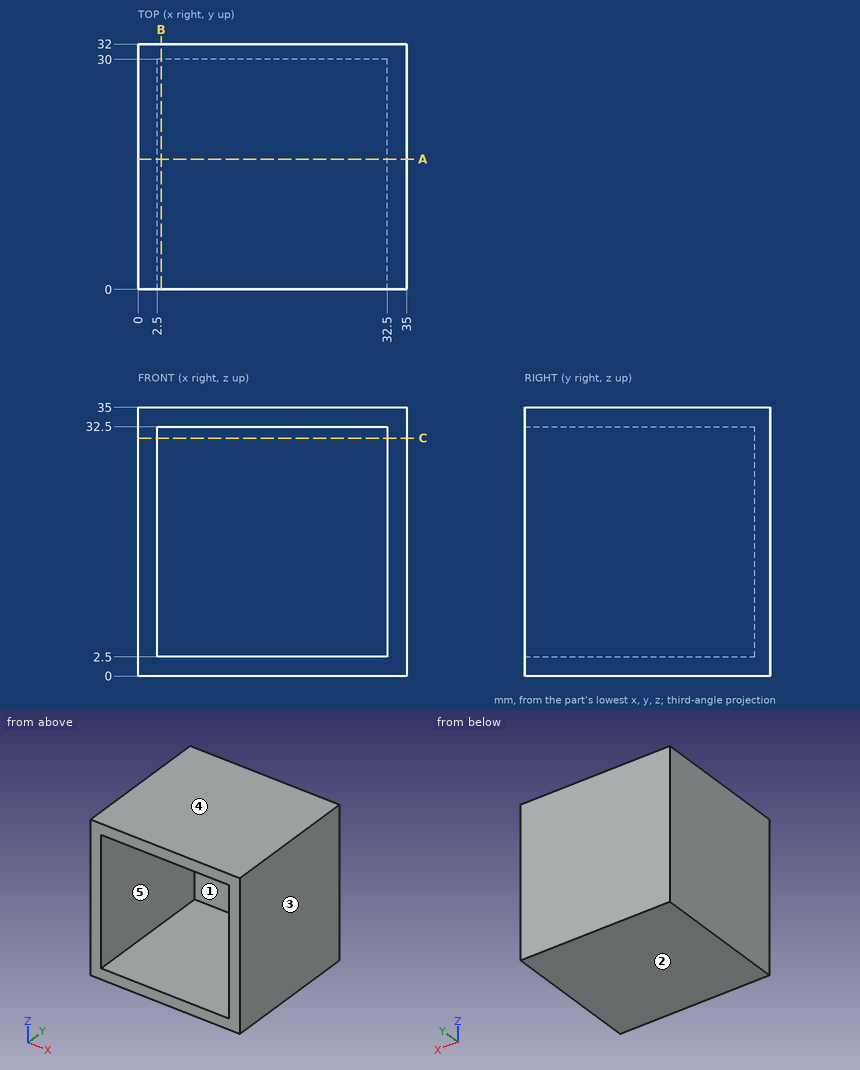
For this review, use the dimensioned drawing (mm, ordinates from the lowest corner) and the shaded views. A direction names the side the tool comes from. Give positions to 0.01 mm unless a question says otherwise; leave off trailing zeros. Write each loop counter-clockwise with the first axis right and the second up, starting at its lowest first coordinate (ties: lowest second). Pieces come first, ordered by that corner, then holes. Notation, with made-up numbers: M 88.5,80 L 146.5,80 A35 ccw 146.5,118 Z; hole C 52.25,61 d3. An arc over 180 degrees is marked long. Answer as a JSON object with one key per item and string values. Group by question number.
1) We need section C-C (z = 31). Give the boundary of the cut face in (x, y), and give its area (3 significant figures).
2) We need section A-A (y = 17). Give the boundary of the cut face in (x, z), and give its area (3 significant figures).
3) We need section B-B (x = 3). Give the boundary of the cut face in (y, z), and give its area (3 significant figures).
4) Mouldability with a two-part tool opening along Z and no side actions: class the marked faces 3, 4 and 5 as released by +Z, released by -Z, zero draft, split by the parting line, or undercut.
5) For line 1 along X through (y, z) = (5, 3.5); line 2 along Y through (x, z) = (22.5, 27), list the stretches that pass through material, from the lowest coordinate up.
6) Tool access review of the marked faces 1 and 2: name each direction out of +Z, -Z, +X, -X, +Y, -Y from which nothing blocks a thin tool from reaching the whole face with its end or side.
7) Clearance check with a flat-ended pin moving along its axis: pin 1 Ø15 at (x, z) = (24, 13.5) entering from -Y. State where the tip first meets the part, or that it passes through.
Answer key:
{
 "1": {"outline": "M 0,0 L 2.5,0 L 2.5,30 L 32.5,30 L 32.5,0 L 35,0 L 35,32 L 0,32 Z", "area": "220 mm²"},
 "2": {"outline": "M 0,0 L 35,0 L 35,35 L 0,35 Z; hole M 2.5,2.5 L 32.5,2.5 L 32.5,32.5 L 2.5,32.5 Z", "area": "325 mm²"},
 "3": {"outline": "M 0,0 L 32,0 L 32,35 L 0,35 L 0,32.5 L 30,32.5 L 30,2.5 L 0,2.5 Z", "area": "220 mm²"},
 "4": {"face 3": "zero draft", "face 4": "released by +Z", "face 5": "undercut"},
 "5": {"line 1": "x = 0 to 2.5, 32.5 to 35", "line 2": "y = 30 to 32"},
 "6": {"face 1": "-Y", "face 2": "-Z, +X, -X, +Y, -Y"},
 "7": {"pin 1": "stops at y = 30"}
}
